The drawing under review shows one solid part. Ordinate dimensions are in mm from its lowest x, y, z. A direction names the side the tool comes from. Coordinates: 2 decimals unless noted, no trailing zeros. Loops run counter-clockwise (first coordinate to the right, second up) from the corner with the lowest first, then second, coordinate; pieces in that order, holes last. Notation, with made-up numbers: (45.5, 49.25) -> (68.5, 49.25) arc R12 cw to (68.5, 66.25) -> close; hole circle Ø11 at (-38.5, 31). An arc over 180 degrees is marked (long way). Use a Markdown table: item, result.
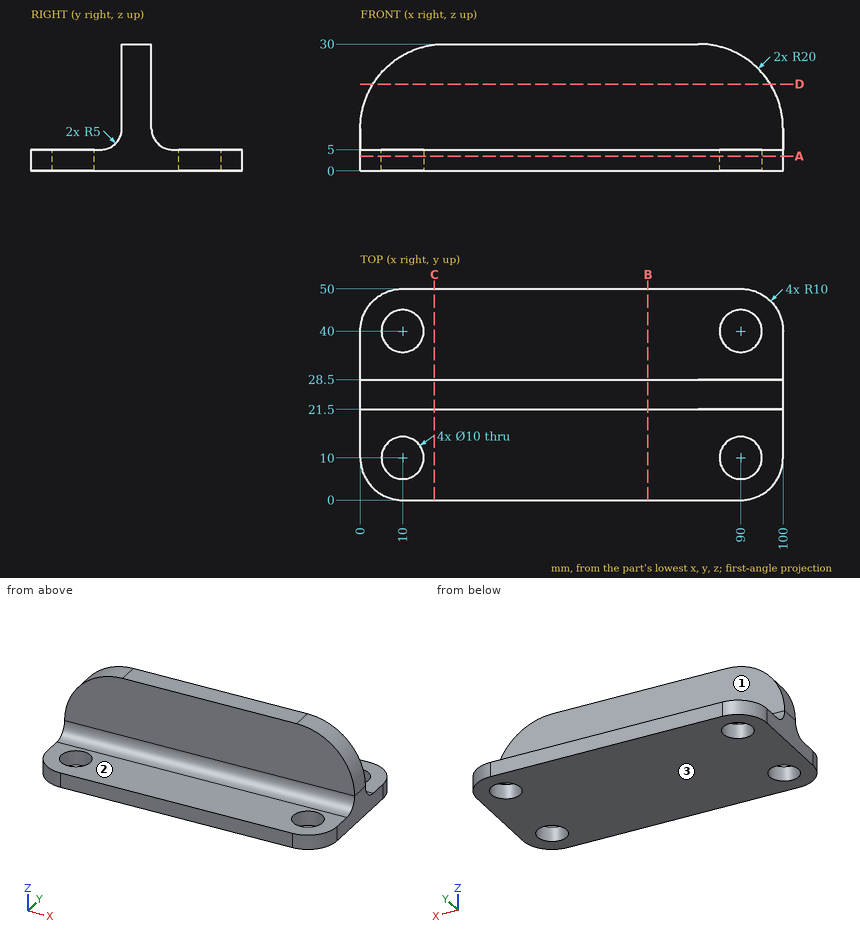
(1) For the marked faces 1, 2 and 3, list the 3-axis set-ups (+Z, -Z, +X, -X, +Y, -Y) from which the entire face can be reached by the end or side of a thin tool; tool diameter is ignored.
Found:
| item | result |
|---|---|
| face 1 | +Z, +X, -X, +Y |
| face 2 | +Z, +X, -X, -Y |
| face 3 | -Z, +X, -X, +Y, -Y |
(2) Take a section at D-D on z = 20.5. Write out the cut boundary in (x, y), plus the area to 3 significant figures.
Found:
| item | result |
|---|---|
| outline | (2.98, 21.5) -> (97.02, 21.5) -> (97.02, 28.5) -> (2.98, 28.5) -> close |
| area | 658 mm^2 |
(3) Take a section at C-C on x = 17.5. Write out the cut boundary in (y, z).
Found:
| item | result |
|---|---|
| outline | (0, 0) -> (50, 0) -> (50, 5) -> (33.5, 5) arc R5 cw to (28.5, 10) -> (28.5, 29.84) -> (21.5, 29.84) -> (21.5, 10) arc R5 cw to (16.5, 5) -> (0, 5) -> close |
(4) Take a section at A-A on z = 3.5. Write out the cut boundary in (x, y).
Found:
| item | result |
|---|---|
| outline | (0, 10) arc R10 ccw to (10, 0) -> (90, 0) arc R10 ccw to (100, 10) -> (100, 40) arc R10 ccw to (90, 50) -> (10, 50) arc R10 ccw to (0, 40) -> close; hole circle Ø10 at (10, 10); hole circle Ø10 at (10, 40); hole circle Ø10 at (90, 10); hole circle Ø10 at (90, 40) |
(5) For pin 1 Ø8 at (x, y) = (10, 10) entering from +Z; pin 2 Ø6 at (x, z) = (48.5, 19.5) entering from +Y; pin 3 Ø5 at (x, y) = (27.5, 40) entering from +Z; pin 4 Ø18 at (x, y) = (32, 12) entering from +Z, all flat-tipped, find the tip position at first contact; note any pin that passes through.
Found:
| item | result |
|---|---|
| pin 1 | passes through |
| pin 2 | stops at y = 28.5 |
| pin 3 | stops at z = 5 |
| pin 4 | stops at z = 7.82 |
(6) Take a section at B-B on x = 68. Write out the cut boundary in (y, z), plus the area to 3 significant figures.
Found:
| item | result |
|---|---|
| outline | (0, 0) -> (50, 0) -> (50, 5) -> (33.5, 5) arc R5 cw to (28.5, 10) -> (28.5, 30) -> (21.5, 30) -> (21.5, 10) arc R5 cw to (16.5, 5) -> (0, 5) -> close |
| area | 436 mm^2 |
(7) For line 1 along Y through (x, z) = (90, 2.6); line 2 along Z through (x, y) = (85, 14); line 3 along Y through (x, z) = (87, 24), list the stretches that pass through material, from the lowest coordinate up.
Found:
| item | result |
|---|---|
| line 1 | y = 0 to 5, 15 to 35, 45 to 50 |
| line 2 | z = 0 to 5 |
| line 3 | y = 21.5 to 28.5 |
